Could you check a few things on this model? Use its own coordinates, in mm. Coordinates: 2 decimals unless noted, no trailing zeros. Order: outer loops, then holes, each group sorted by start corner. A loop starts at its lowest first (then second) coordinate and runs counter-clockwise, first axis right, second up. Notation, with made-up numbers: (41, 63) -> (79, 63) arc R25 cw to (79, 82) -> close; hole circle Ø6 at (-10.5, 23.25). An arc over 180 degrees is marked (long way). Return JSON: item names as keys, results as strings. Group by question number.
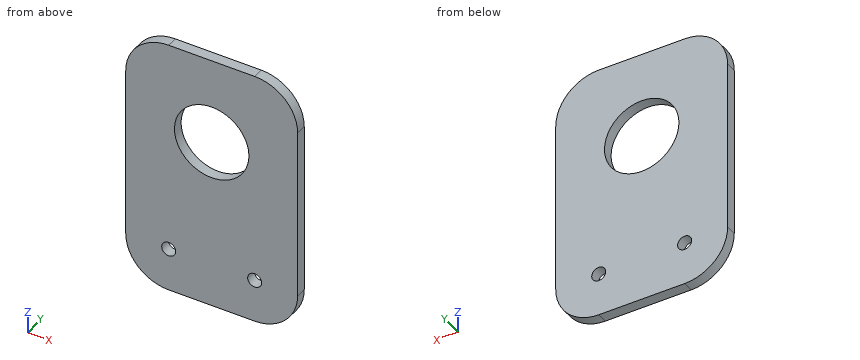
Autodesk Inventor part; units mm, degrees
ref_plane "YZ Plane" through (0, 0, 0) normal (1, 0, 0) x (0, 1, 0)
ref_plane "XZ Plane" through (0, 0, 0) normal (0, 1, 0) x (-1, 0, 0)
ref_plane "XY Plane" through (0, 0, 0) normal (0, 0, 1) x (1, 0, 0)
sketch "Sketch1" plane through (0, 0, 0) normal (0, 0, 1) x (1, 0, 0)
  line L0 (-25.4, -1.5875) -> (25.4, -1.5875)
  line L1 (25.4, -1.5875) -> (25.4, 1.5875)
  line L2 (25.4, 1.5875) -> (-25.4, 1.5875)
  line L3 (-25.4, 1.5875) -> (-25.4, -1.5875)
  line L4 (-25.4, -1.5875) -> (25.4, 1.5875) construction
  line L5 (25.4, -1.5875) -> (-25.4, 1.5875) construction
  point P0 (0, 0)
  dimension "d0" = 3.175
  dimension "d1" = 50.8
extrude "Extrusion1" add sketch "Sketch1" along normal blind 76.2
sketch "Sketch2" plane through (-25.4, 1.5875, 0) normal (0, 1, 0) x (1, 0, 0)
  line L0 (50.8, 0) -> (50.8, -76.2)
  line L1 (0, 0) -> (0, -76.2)
  line L2 (50.8, 0) -> (0, 0)
  line L3 (50.8, -76.2) -> (0, -76.2)
  point P0 (25.4, 0)
  point P1 (38.1, -12.7)
  point P2 (12.7, -12.7)
  point P3 (25.4, -50.8)
  dimension "d4" = 12.7
  dimension "d5" = 12.7
  dimension "d6" = 12.7
  dimension "d7" = 12.7
  dimension "d8" = 25.4
  dimension "d9" = 25.4
hole "Hole1" at (12.7, 1.5875, 12.7) at (-12.7, 1.5875, 12.7) direction (0, -1, 0) diameter 4.1402 end through all
hole "Hole2" at (0, 1.5875, 50.8) direction (0, -1, 0) diameter 22 end through all
fillet "Fillet1" radius 12.7 4 edges at (-25.4, 0, 0) (25.4, 0, 0) (25.4, 0, 76.2) (-25.4, 0, 76.2)
properties part number "C33_TK_IdiotLightBracket" material "Polycarbonate, Clear"
Q1. I need wall thicknesses on line 1 along X through (y, z) = (-0.25, 12.7); line 2 along Z through (x, y) = (0, -0.25); line 3 along X through (y, z) = (1.3, 12). Which ranges of each line are inside material? Lowest first, please. Write a range as from..to.
Q2. I want a section at D-D on x = 18. Please give me the cut outline in (y, z), and give its area (3 significant figures).
Q3. I want a section at B-B on x = 0. Please give me the cut outline in (y, z), and give its area (3 significant figures).
Q4. I want a section at A-A on z = 50.8. Please give me the cut outline in (x, y), and give its area (3 significant figures).
Q5. I want a section at C-C on y = 0.5. Please give me the cut outline in (x, z).
Q6. I'm going to push flat-ended pins straight in: pin 1 Ø17.5 at (x, z) = (0, 50.8) entering from +Y; pin 2 Ø5.5 at (x, z) = (12.7, 12.7) entering from -Y. Where does each tip first touch, or does it pass through?
Response values:
{
 "1": {"line 1": "x = -25.4..-14.77, -10.63..10.63, 14.77..25.4", "line 2": "z = 0..39.8, 61.8..76.2", "line 3": "x = -25.38..-14.65, -10.75..10.75, 14.65..25.38"},
 "2": {"outline": "(-1.59, 1.16) -> (1.59, 1.16) -> (1.59, 75.04) -> (-1.59, 75.04) -> close", "area": "235 mm²"},
 "3": {"outline": "(-1.59, 0) -> (1.59, 0) -> (1.59, 39.8) -> (-1.59, 39.8) -> close; (-1.59, 61.8) -> (1.59, 61.8) -> (1.59, 76.2) -> (-1.59, 76.2) -> close", "area": "172 mm²"},
 "4": {"outline": "(-25.4, -1.59) -> (-11, -1.59) -> (-11, 1.59) -> (-25.4, 1.59) -> close; (11, -1.59) -> (25.4, -1.59) -> (25.4, 1.59) -> (11, 1.59) -> close", "area": "91.4 mm²"},
 "5": {"outline": "(-25.4, 12.7) arc R12.7 ccw to (-12.7, 0) -> (12.7, 0) arc R12.7 ccw to (25.4, 12.7) -> (25.4, 63.5) arc R12.7 ccw to (12.7, 76.2) -> (-12.7, 76.2) arc R12.7 ccw to (-25.4, 63.5) -> close; hole circle Ø4.14 at (-12.7, 12.7); hole circle Ø22 at (0, 50.8); hole circle Ø4.14 at (12.7, 12.7)"},
 "6": {"pin 1": "passes through", "pin 2": "stops at y = -1.59"}
}
